Autodesk Inventor part; units mm, degrees
ref_plane "YZ Plane" through (0, 0, 0) normal (1, 0, 0) x (0, 1, 0)
ref_plane "XZ Plane" through (0, 0, 0) normal (0, 1, 0) x (-1, 0, 0)
ref_plane "XY Plane" through (0, 0, 0) normal (0, 0, 1) x (1, 0, 0)
ref_plane "Arbeitsebene1" through (0, 0, 0) normal (0, 0, 1) x (1, 0, 0)
sketch "Skizze1" plane through (0, 0, 0) normal (0, 0, 1) x (1, 0, 0)
  line L0 (14.5712, 11.3758) -> (14.5712, 4.0068)
  line L1 (13.3638, -15.5) -> (13.3638, 1.7)
  arc A0 (14.5712, 4.0068) -> (13.3638, 1.7) centre (16.1712, 1.7) ccw
  line L2 (8.0712, 15) -> (38.0712, 15)
  line L3 (38.0712, 15) -> (38.0712, -15)
  line L4 (38.0712, -15) -> (8.0712, -15)
  line L5 (8.0712, -15) -> (8.0712, 15)
  line L6 (38.0712, 19) -> (8.0712, 19)
  line L7 (4.0712, 15) -> (4.0712, -15)
  line L8 (8.0712, -19) -> (38.0712, -19)
  line L9 (42.0712, -15) -> (42.0712, 15)
  arc A1 (8.0712, 19) -> (4.0712, 15) centre (8.0712, 15) ccw
  arc A2 (42.0712, 15) -> (38.0712, 19) centre (38.0712, 15) ccw
  arc A3 (38.0712, -19) -> (42.0712, -15) centre (38.0712, -15) ccw
  arc A4 (4.0712, -15) -> (8.0712, -19) centre (8.0712, -15) ccw
  line L10 (10.5793, 11.3758) -> (14.5712, 11.3758)
  line L11 (36.5793, 10.3758) -> (36.5793, -24.4)
  arc A5 (36.5793, 10.3758) -> (35.5793, 11.3758) centre (35.5793, 10.3758) ccw
  line L12 (9.5793, -24.4) -> (9.5793, 10.3758)
  line L13 (36.5793, -24.4) -> (9.5793, -24.4)
  line L14 (31.5712, 11.3758) -> (35.5793, 11.3758)
  line L15 (31.5712, 4.0068) -> (31.5712, 11.3758)
  arc A6 (10.5793, 11.3758) -> (9.5793, 10.3758) centre (10.5793, 10.3758) ccw
  arc A7 (32.7786, 1.7) -> (31.5712, 4.0068) centre (29.9712, 1.7) ccw
  line L16 (32.7786, 1.7) -> (32.7786, -15.5)
  arc A8 (29.9712, -18.3074) -> (32.7786, -15.5) centre (29.9712, -15.5) ccw
  line L17 (29.9712, -18.3074) -> (16.1712, -18.3074)
  arc A9 (13.3638, -15.5) -> (16.1712, -18.3074) centre (16.1712, -15.5) ccw
  point P0 (0, 0)
  dimension "d0" = 4
  dimension "d1" = 4
extrude "Extrusion1" add sketch "Skizze1" along normal blind 2 contours L10 A6 L12 L4 L5 L2 L3 L11 A5 L14 L15 A7 L16 L1 A0 L0 | L0 A0 L1 L4 L12 A6 L10 | L4 L16 A8 L17 A9 L1 | L1 A9 L17 A8 L16 L4 L11 L8 L12 | L12 L8 A4 L7 A1 L6 A2 L9 A3 L11 L4 L3 L2 L5 | L16 A7 L15 L14 A5 L11 L4
ref_plane "Arbeitsebene2" through (0, 0, 0) normal (0, 0, 1) x (1, 0, 0)
sketch "Skizze2" plane through (0, 0, 2) normal (0, 0, 1) x (1, 0, 0)
  arc A0 (8.0712, 19) -> (4.0712, 15) centre (8.0712, 15) ccw
  line L0 (4.0712, 15) -> (4.0712, -15)
  arc A1 (4.0712, -15) -> (8.0712, -19) centre (8.0712, -15) ccw
  line L1 (8.0712, -19) -> (38.0712, -19)
  arc A2 (38.0712, -19) -> (42.0712, -15) centre (38.0712, -15) ccw
  line L2 (42.0712, -15) -> (42.0712, 15)
  arc A3 (42.0712, 15) -> (38.0712, 19) centre (38.0712, 15) ccw
  line L3 (38.0712, 19) -> (8.0712, 19)
  circle A4 centre (8.0712, 15) radius 1.4
  circle A5 centre (38.0712, 15) radius 1.4
  circle A6 centre (38.0712, -15) radius 1.4
  circle A7 centre (8.0712, -15) radius 1.4
  point P0 (0, 0)
hole "Bohrung1" at (8.0712, 15, 2) at (8.0712, -15, 2) at (38.0712, -15, 2) at (38.0712, 15, 2) direction (0, 0, -1) diameter 3.2 end through all
properties part number "20_Cube_Insert_SEEED_Xiao_Sense_Camera_backplate"
Here's how the part is built. I have some questions about the finished solid (model axes, mm). Give positions to 0.01 mm unless a question says otherwise; leave off trailing zeros. Write each loop counter-clockwise with the first axis right and the second up, starting at its lowest first coordinate (ties: lowest second). Pieces come first, ordered by that corner, then holes. Notation, with made-up numbers: M 31.25,58 L 78.25,58 A3 ccw 78.25,63 Z; hole C 68,37.25 d1. An arc over 180 degrees is marked long. Put each result on its own line as item: value. Start each with the question number.
Item 1: Will this pin go through, and if not, where does the flat tip stop? pin 1 (1.9 mm diameter, centred on x = 8.07, y = -15, fed in from -Z).
Item 2: Thinking about a two-plate mould opening in Y: for faces 1 (the flat face through (23, 19, 1)), 2 (the cylindrical face through (36.99, 16.18, 0.99)), 3 (the flat face through (4.071, 0, 1)), which applies, +Y half, -Y half, draft (parallel to the pull), parting line (faces both ways), or undercut?
Item 3: If we section it at B-B, the plane x = 7.5: Write out the boundary of the cut face in (y, z), then the cut area to 3 significant figures.
Item 4: If we section it at A-A, the plane z = 1.7: Write out the boundary of the cut face in (x, y), then the cut area to 3 significant figures.
Item 5: I need wall thicknesses on L1, parallel to Y at x = 38, z = 1.8; L2, parallel to X at y = 15, z = 1.6; L3, parallel to X at y = 17, z = 1.65. Which ranges of each line are inside material? Lowest first, please. Write a range as from..to.
Values:
1. pin 1: through
2. face 1: +Y half
2. face 2: undercut
2. face 3: draft
3. outline: M -18.96,0 L -16.49,0 L -16.49,2 L -18.96,2 Z; M -13.51,0 L 13.51,0 L 13.51,2 L -13.51,2 Z; M 16.49,0 L 18.96,0 L 18.96,2 L 16.49,2 Z
3. area: 63.9 mm²
4. outline: M 4.07,-15 A4 ccw 8.07,-19 L 38.07,-19 A4 ccw 42.07,-15 L 42.07,15 A4 ccw 38.07,19 L 8.07,19 A4 ccw 4.07,15 Z; hole C 8.07,-15 d3.2; hole C 8.07,15 d3.2; hole C 38.07,-15 d3.2; hole C 38.07,15 d3.2
4. area: 1,400 mm²
5. L1: -19..-16.6, -13.4..13.4, 16.6..19
5. L2: 4.07..6.47, 9.67..36.47, 39.67..42.07
5. L3: 4.61..41.54
